Geometry: see drawing. Coordinates: mm, zero at the bounding-box minimum. A direction names the side the tool comes from. Round coordinates to 2 decimals unless told otherwise and drop trailing zeros. Write each loop counter-clockwise with the first axis right and the second up, starting at its lowest first coordinate (ties: lowest second). Pieces come first, ordered by that corner, then holes.
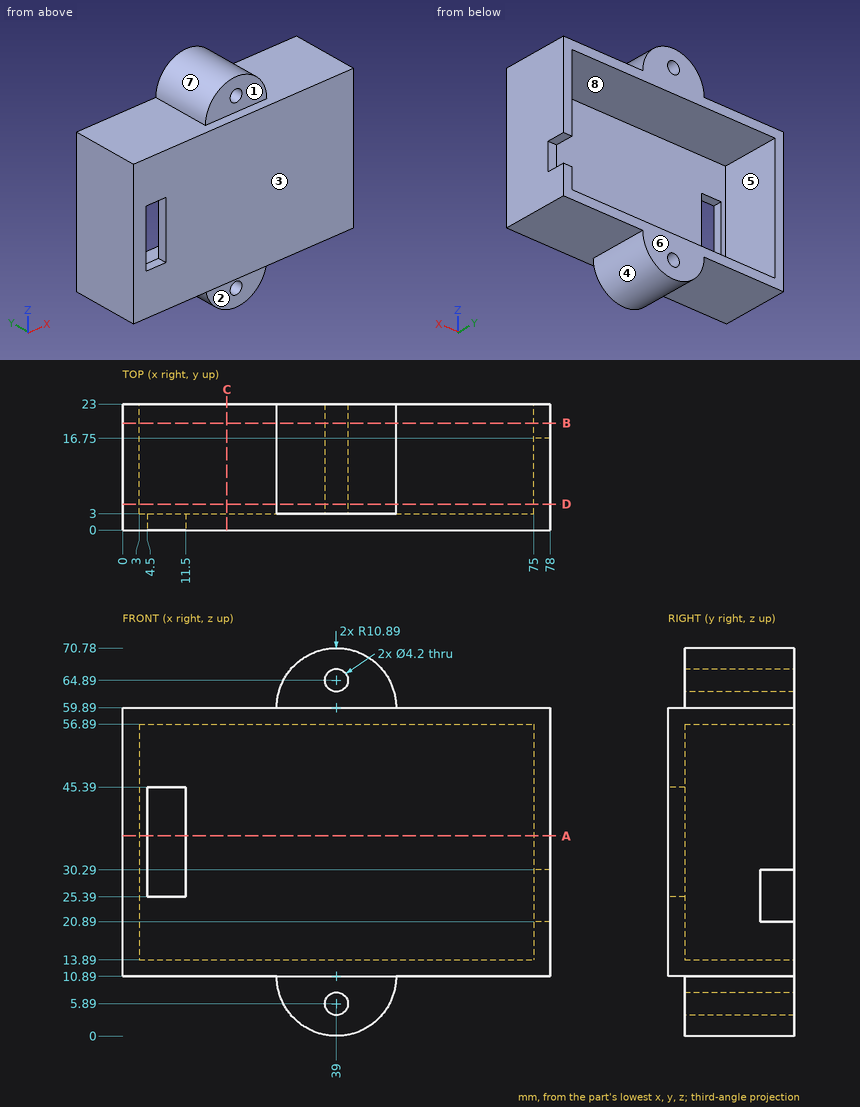
1) Pull-direction query (X, two-part tool) for the marked faces 6, 7 and 8; classes: released by +X, released by -X, zero draft, split by the parting line, or undercut.
Taken from the geometry:
face 6: zero draft
face 7: split by the parting line
face 8: undercut
2) Material intervals for line 1 (Z direction, x = 10, y = 7.5); line 2 (X direction, y = 19.75, z = 53); line 3 (Y direction, x = 57, z = 40), sorted ascending.
Taken from the geometry:
line 1: z = 10.89 to 13.89, 56.89 to 59.89
line 2: x = 0 to 3, 75 to 78
line 3: y = 0 to 3
3) Section query C-C on x = 19. Return the cut outline in (y, z), then the cut area to 3 significant figures.
Taken from the geometry:
outline: (0, 10.89) - (23, 10.89) - (23, 13.89) - (3, 13.89) - (3, 56.89) - (23, 56.89) - (23, 59.89) - (0, 59.89) - close
area: 267 mm2
4) Section query A-A on z = 36.5. Return the cut outline in (x, y).
Taken from the geometry:
outline: (0, 0) - (4.5, 0) - (4.5, 3) - (3, 3) - (3, 23) - (0, 23) - close; (11.5, 0) - (78, 0) - (78, 23) - (75, 23) - (75, 3) - (11.5, 3) - close
5) Section query B-B on y = 19.5. Return the cut outline in (x, z), then the cut area to 3 significant figures.
Taken from the geometry:
outline: (0, 10.89) - (28.11, 10.89) arc R10.89 ccw to (49.89, 10.89) - (78, 10.89) - (78, 20.89) - (75, 20.89) - (75, 13.89) - (3, 13.89) - (3, 56.89) - (75, 56.89) - (75, 30.29) - (78, 30.29) - (78, 59.89) - (49.89, 59.89) arc R10.89 ccw to (28.11, 59.89) - (0, 59.89) - close; hole circle Ø4.2 at (39, 5.89); hole circle Ø4.2 at (39, 64.89)
area: 1,040 mm2
6) Reachability of the marked faces 1, 2, 3, 4 and 5 from +Z, -Z, +X, -X, +Y, -Y: full face, straight path, thin tool, end or side. Return the list, or none.
Taken from the geometry:
face 1: +Z, +X, -X, -Y
face 2: -Z, +X, -X, -Y
face 3: +Z, -Z, +X, -X, -Y
face 4: -Z, +Y, -Y
face 5: +Y
7) Section query D-D on y = 4.75. Return the cut outline in (x, z), then the cut area to 3 significant figures.
Taken from the geometry:
outline: (0, 10.89) - (28.11, 10.89) arc R10.89 ccw to (49.89, 10.89) - (78, 10.89) - (78, 59.89) - (49.89, 59.89) arc R10.89 ccw to (28.11, 59.89) - (0, 59.89) - close; hole (3, 13.89) - (75, 13.89) - (75, 56.89) - (3, 56.89) - close; hole circle Ø4.2 at (39, 5.89); hole circle Ø4.2 at (39, 64.89)
area: 1,070 mm2
8) Contact query for flat-ended pins moving along their axis: P1, Ø10, axis at y = 11, z = 36, coming from the -X side; P2, Ø3.5, axis at x = 76, y = 19, coming from the +Z side; P3, Ø0.9, axis at x = 76.5, y = 19, coming from the -Z side; P4, Ø1.5, axis at x = 20.5, z = 54, coming from the +Y side. Output: stop coordinate, or through.
Taken from the geometry:
P1: stops at x = 0
P2: stops at z = 59.89
P3: stops at z = 10.89
P4: stops at y = 3
